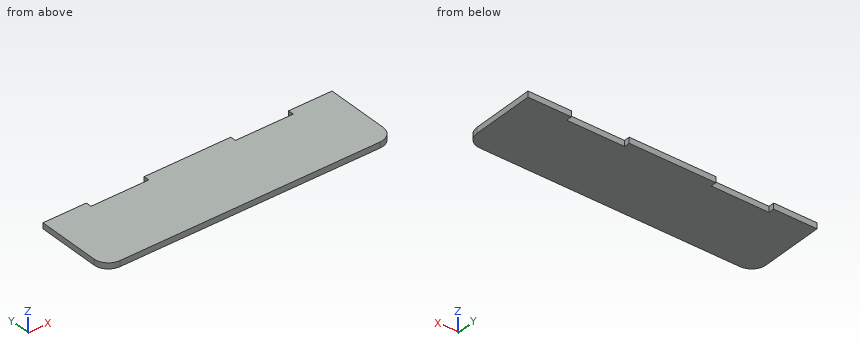
from build123d import *

# Parameters (mm, degrees)
BOSS_EXTRUDE1_DEPTH = 4


with BuildPart() as part:
    # Sketch1 → Boss-Extrude1 (new body)
    with BuildSketch(Plane.XY):
        with BuildLine():
            Line((10, 0), (190, 0))
            ThreePointArc((190, 0), (197.071067812, 2.928932188), (200, 10))
            Line((200, 10), (200, 50))
            Line((200, 50), (200, 54))
            Line((200, 54), (170, 54))
            Line((170, 54), (170, 50))
            Line((170, 50), (130, 50))
            Line((130, 50), (130, 54))
            Line((130, 54), (70, 54))
            Line((70, 54), (70, 50))
            Line((70, 50), (30, 50))
            Line((30, 50), (30, 54))
            Line((30, 54), (0, 54))
            Line((0, 54), (0, 50))
            Line((0, 50), (0, 10))
            ThreePointArc((0, 10), (2.928932188, 2.928932188), (10, 0))
        make_face()
    extrude(amount=BOSS_EXTRUDE1_DEPTH)


solid = part.part
Build history of the part. All positions in model axes, mm. Coordinates: 2 decimals unless noted, no trailing zeros. Order: outer loops, then holes, each group sorted by start corner. A loop starts at its lowest first (then second) coordinate and runs counter-clockwise, first axis right, second up. Notation, with made-up numbers: M 20,-2 L 32,-2 A21 cw 32,5 Z; hole C -11.75,88.5 d2. An arc over 180 degrees is marked long. One line per question, with ' | ' between items. Start each with the question number.
Q1. Probe L1, parallel to Y at x = 131.5, z = 1.8; L2, parallel to X at y = 3, z = 2.15; L3, parallel to X at y = 8.5, z = 1.4. List the from-to ranges inside material, lowest first. Write a range as from..to.
Q2. Saw through at B-B (x = 167). List the corners of the cut face in (y, z), then the cut area to 3 significant figures.
Q3. Saw through at A-A (z = 3.3). List the corners of the cut face in (x, y), then the cut area to 3 significant figures.
Q4. Flat gauge pin, fed straight in: pin 1 Ø1.2 at (x, z) = (52.5, 2.5) entering from +Y. Where does the tip first touch, or does it go through?
Check values:
1) L1: y = 0..50 | L2: x = 2.86..197.14 | L3: x = 0.11..199.89
2) outline: M 0,0 L 50,0 L 50,4 L 0,4 Z | area: 200 mm2
3) outline: M 0,10 A10 ccw 10,0 L 190,0 A10 ccw 200,10 L 200,54 L 170,54 L 170,50 L 130,50 L 130,54 L 70,54 L 70,50 L 30,50 L 30,54 L 0,54 Z | area: 10,400 mm2
4) pin 1: stops at y = 50
